Read the model definition and answer for the solid it produces. Units are mm, in the model's axes. A direction names the side the tool comes from. Round coordinates to 2 decimals unless told otherwise and drop trailing zeros. Loops run counter-clockwise (first coordinate to the right, second up) from the corner with the lowest first, then second, coordinate; pieces in that order, holes last. Notation, with made-up numbers: (-33, 65.5) - (9, 65.5) arc R20 cw to (9, 78.5) - close; hole circle Ø10 at (6, 74). An arc over 180 degrees is marked (long way). Answer as CSV lines item,"result".
Autodesk Inventor part; units mm, degrees
ref_plane "YZ Plane" through (0, 0, 0) normal (1, 0, 0) x (0, 1, 0)
ref_plane "XZ Plane" through (0, 0, 0) normal (0, 1, 0) x (-1, 0, 0)
ref_plane "XY Plane" through (0, 0, 0) normal (0, 0, 1) x (1, 0, 0)
sketch "Sketch1" plane through (0, 0, 0) normal (0, 1, 0) x (-1, 0, 0)
  line L0 (35, 50) -> (-35, 50)
  line L1 (-35, 50) -> (-35, -50)
  line L2 (-35, -50) -> (35, -50)
  line L3 (35, -50) -> (35, 50)
  line L4 (35, 50) -> (-35, -50) construction
  line L5 (-35, 50) -> (35, -50) construction
  point P0 (0, 0)
  dimension "d0" = 100
  dimension "d1" = 70
extrude "Extrusion1" add sketch "Sketch1" along normal blind 5
sketch "Sketch2" plane through (0, 5, 0) normal (0, 1, 0) x (1, 0, 0)
  line L0 (30, 45) -> (30, -7)
  line L1 (-18, 45) -> (30, 45)
  line L2 (-35, -50) -> (35, -50)
  line L3 (35, -50) -> (35, 50)
  arc A0 (-18, 45) -> (-30, 33) centre (-18, 33) ccw
  line L4 (-30, 33) -> (-30, 0)
  line L5 (-30, 0) -> (-20, -45)
  arc A1 (-12, -45) -> (3, -30) centre (-12, -30) ccw
  line L6 (-20, -45) -> (-12, -45)
  line L7 (3, -30) -> (3, -25)
  arc A2 (11, -17) -> (3, -25) centre (11, -25) ccw
  arc A3 (20, -17) -> (30, -7) centre (20, -7) ccw
  line L8 (11, -17) -> (20, -17)
  point P0 (0, 0)
  dimension "d4" = 95
  dimension "d5" = 5
  dimension "d6" = 24
  dimension "d7" = 65
  dimension "d8" = 50
  dimension "d9" = 55
  dimension "d10" = 5
  dimension "d11" = 30
  dimension "d12" = 32
  dimension "d13" = 16
  dimension "d15" = 20
extrude "Extrusion2" add sketch "Sketch2" along normal blind 5
sketch "Sketch3" plane through (0, 10, 0) normal (0, 1, 0) x (1, 0, 0)
  line L0 (-22, 1.52) -> (-10, 1.52)
  line L1 (-6, 5.52) -> (-6, 32.52)
  line L2 (-10, 36.52) -> (-22, 36.52)
  line L3 (-26, 32.52) -> (-26, 5.52)
  line L4 (-23.2444, 1.52) -> (-8.7556, 34.48) construction
  line L5 (-6.9662, 2.9131) -> (-22.5304, 28.9061) construction
  arc A0 (-6, 32.52) -> (-10, 36.52) centre (-10, 32.52) ccw
  arc A1 (-22, 36.52) -> (-26, 32.52) centre (-22, 32.52) ccw
  arc A2 (-26, 5.52) -> (-22, 1.52) centre (-22, 5.52) ccw
  arc A3 (-10, 1.52) -> (-6, 5.52) centre (-10, 5.52) ccw
  line L6 (35, -50) -> (35, 50)
  line L7 (-35, -50) -> (35, -50)
  line L8 (15, 26) -> (15, 11)
  line L9 (30, 7) -> (30, 30)
  line L10 (30, 30) -> (15, 7) construction
  line L11 (15, 30) -> (30, 7) construction
  line L12 (30, -7) -> (30, 45)
  arc A4 (19, 30) -> (15, 26) centre (19, 26) ccw
  arc A5 (15, 11) -> (19, 7) centre (19, 11) ccw
  line L13 (30, 34) -> (17.7027, 29.7838)
  line L14 (30, 3) -> (17.7027, 7.2162)
  line L15 (30, 7) -> (30, 3)
  line L16 (30, 34) -> (30, 30)
  point P0 (0, 0)
  point P1 (-16, 18)
  point P2 (-26, 19.02)
  point P3 (-16, 36.52)
  point P4 (22.5, 18.5)
  point P5 (22.5, 7)
  dimension "d18" = 8
  dimension "d19" = 8
  dimension "d20" = 8
  dimension "d22" = 8
  dimension "d23" = 35
  dimension "d24" = 20
  dimension "d25" = 51
  dimension "d26" = 68
  dimension "d27" = 51
  dimension "d28" = 20
  dimension "d29" = 0
  dimension "d32" = 8
  dimension "d33" = 8
  dimension "d34" = 84
  dimension "d35" = 53
extrude "Extrusion3" cut sketch "Sketch3" against normal blind 4
sketch "Sketch4" plane through (0, 10, 0) normal (0, 1, 0) x (1, 0, 0)
  circle A0 centre (5, -5) radius 4
  circle A1 centre (5, 10) radius 4
  circle A2 centre (5, 25) radius 4
  line L0 (-35, -50) -> (35, -50)
  line L1 (35, -50) -> (35, 50)
  point P0 (0, 0)
  dimension "d38" = 8
  dimension "d39" = 8
  dimension "d40" = 8
  dimension "d41" = 45
  dimension "d42" = 60
  dimension "d43" = 75
  dimension "d44" = 30
  dimension "d45" = 30
  dimension "d46" = 30
extrude "Extrusion4" cut sketch "Sketch4" against normal blind 2
properties part number "Exercise4"
1) Each of these flat-tipped pins is pushed along its axis until it touches: P1, Ø2.5, axis at x = -4, y = 7, coming from the -Z side; P2, Ø3, axis at x = -14.5, y = 8.5, coming from the +Z side; P3, Ø2, axis at x = 4, z = -26, coming from the +Y side. Where does it stop, or does it pass through?
Entries:
P1,"stops at z = -45"
P2,"stops at z = 45"
P3,"stops at y = 8"
2) Find the intervals of material crossed by line 1 (X direction, y = 8.75, z = -25); line 2 (Z direction, x = 5, y = 9.45); line 3 (Y direction, x = 5, z = 42), in increasing order.
Entries:
line 1,"x = -30 to -26, -6 to 1, 9 to 15"
line 2,"z = -45 to -29, -21 to -14, -6 to 1, 9 to 19.71"
line 3,"y = 0 to 5"
3) A cutting plane is placed at A-A, the plane x = 13. Determine the outline of the cut face in (y, z).
Entries:
outline,"(0, -50) - (5, -50) - (5, -45) - (10, -45) - (10, 17) - (5, 17) - (5, 50) - (0, 50) - close"
4) A cutting plane is placed at D-D, the plane x = 5. Determine the outline of the cut face in (y, z).
Entries:
outline,"(0, -50) - (5, -50) - (5, -45) - (10, -45) - (10, -29) - (8, -29) - (8, -21) - (10, -21) - (10, -14) - (8, -14) - (8, -6) - (10, -6) - (10, 1) - (8, 1) - (8, 9) - (10, 9) - (10, 19.71) - (5, 19.71) - (5, 50) - (0, 50) - close"
5) A cutting plane is placed at B-B, the plane z = -25. Determine the outline of the cut face in (x, y).
Entries:
outline,"(-35, 0) - (35, 0) - (35, 5) - (30, 5) - (30, 6) - (15, 6) - (15, 10) - (9, 10) - (9, 8) - (1, 8) - (1, 10) - (-6, 10) - (-6, 6) - (-26, 6) - (-26, 10) - (-30, 10) - (-30, 5) - (-35, 5) - close"
6) A tool of negligible diameter and unlimited length cuts with its end or side. For faces 1 (the face through (5, 8, -25)), 2 (the face through (3, 7, 28)), 3 (the face through (-30, 7, -17)), 4 (the face through (-26.58, 7.46, -41.39)), 5 (the face through (23.937, 8.028, -5.079)), from which of +Z, -Z, +X, -X, +Y, -Y can it reach the whole face along a straight path? Write none if from no direction.
Entries:
face 1,"+Y"
face 2,"+Z, +X, +Y"
face 3,"+Z, -Z, -X, +Y"
face 4,"-Z, -X, +Y"
face 5,"+X, +Y"
7) The mould has two halves that part along Z. Classify faces 6 (the face through (0, 2, -50)), 7 (the face through (-25.07, 7.46, 22.18)), 8 (the face through (-24.797, 8.028, -35.379)): pulls with the +Z half, pulls with the -Z half, needs draft (parallel to the pull), parting line crosses it, or undercut.
Entries:
face 6,"pulls with the -Z half"
face 7,"pulls with the +Z half"
face 8,"undercut"
8) A cutting plane is placed at C-C, the plane z = 41. Determine the outline of the cut face in (x, y), plus the area to 3 significant figures.
Entries:
outline,"(-35, 0) - (35, 0) - (35, 5) - (-1.8, 5) - (-1.8, 10) - (-20.89, 10) - (-20.89, 5) - (-35, 5) - close"
area,"445 mm^2"
